Autodesk Inventor part; units mm, degrees
ref_plane "YZ Plane" through (0, 0, 0) normal (1, 0, 0) x (0, 1, 0)
ref_plane "XZ Plane" through (0, 0, 0) normal (0, 1, 0) x (-1, 0, 0)
ref_plane "XY Plane" through (0, 0, 0) normal (0, 0, 1) x (1, 0, 0)
sketch "Sketch1" plane through (0, 0, 0) normal (0, 0, 1) x (1, 0, 0)
  spline S0 degree 3 poles (-37.25, 0) (-37.25, -7.0376) (-35.2039, -14.0633) (-31.4252, -20.0004) (-27.6466, -25.9375) (-22.1482, -30.766) (-15.7726, -33.7459) (-9.397, -36.7258) (-2.1659, -37.8471) (4.8127, -36.9378) (11.7914, -36.0285) (18.4938, -33.0918) (23.893, -28.5778) (29.2921, -24.0637) (33.3697, -17.9875) (35.5009, -11.2804) (37.6321, -4.5732) (37.8097, 2.7422) (36.0064, 9.5448) (34.2031, 16.3475) (30.4251, 22.6143) (25.2512, 27.385) (20.0774, 32.1557) (13.5254, 35.414) (6.5991, 36.6608) (-0.3272, 37.9076) (-7.6042, 37.1385) (-14.1169, 34.4714) (-20.6295, 31.8043) (-26.3557, 27.2483) (-30.4179, 21.5014) (-34.4802, 15.7546) (-36.8647, 8.8365) (-37.2061, 1.8072) (-37.2354, 1.2052) (-37.25, 0.6026) (-37.25, 0) knots 0 0 0 0 0.566787 0.566787 0.566787 1.133573 1.133573 1.133573 1.70036 1.70036 1.70036 2.267146 2.267146 2.267146 2.833933 2.833933 2.833933 3.400719 3.400719 3.400719 3.967506 3.967506 3.967506 4.534292 4.534292 4.534292 5.101079 5.101079 5.101079 5.667865 5.667865 5.667865 6.234652 6.234652 6.234652 6.283185 6.283185 6.283185 6.283185
  spline S1 degree 5 poles (-38.75, 0) (-38.7501, -2.7047) (-38.5078, -5.4094) (-38.0316, -8.0852) (-36.6239, -13.33) (-34.3392, -18.2559) (-32.9845, -20.6148) (-29.8595, -25.0561) (-26.0175, -28.8925) (-23.9357, -30.6396) (-19.4934, -33.7614) (-14.5735, -36.0618) (-12.0149, -36.9831) (-6.7678, -38.3822) (-1.3581, -38.8593) (1.3604, -38.8675) (6.7714, -38.3973) (12.0133, -36.9798) (14.5666, -36.049) (19.4877, -33.7543) (23.9437, -30.6512) (26.0275, -28.9023) (29.8573, -25.0529) (32.972, -20.6052) (34.3321, -18.2523) (36.6385, -13.3362) (38.0403, -8.0889) (38.5046, -5.4103) (38.9743, 0) (38.5079, 5.4103) (38.0448, 8.0901) (36.6331, 13.3345) (34.3305, 18.2516) (32.9714, 20.6051) (29.8608, 25.0551) (26.0293, 28.9037) (23.9413, 30.647) (19.4872, 33.7528) (14.5665, 36.0499) (12.0141, 36.984) (6.7708, 38.3997) (1.3596, 38.8619) (-1.3583, 38.8577) (-6.7678, 38.3823) (-12.0157, 36.988) (-14.5739, 36.063) (-19.4902, 33.7565) (-23.9357, 30.6394) (-26.0178, 28.8927) (-29.8639, 25.0602) (-32.9831, 20.614) (-34.3346, 18.2543) (-36.6237, 13.3303) (-38.0331, 8.0858) (-38.5138, 5.4104) (-38.7506, 2.7047) (-38.75, 0) knots 0 0 0 0 0 0 0.055551 0.055551 0.055551 0.111119 0.111119 0.111119 0.166658 0.166658 0.166658 0.222223 0.222223 0.222223 0.277783 0.277783 0.277783 0.333326 0.333326 0.333326 0.388895 0.388895 0.388895 0.444438 0.444438 0.444438 0.499998 0.499998 0.499998 0.555563 0.555563 0.555563 0.611102 0.611102 0.611102 0.66667 0.66667 0.66667 0.722222 0.722222 0.722222 0.777772 0.777772 0.777772 0.83334 0.83334 0.83334 0.88888 0.88888 0.88888 0.944445 0.944445 0.944445 1 1 1 1 1 1
  spline S2 degree 5 poles (-43.75, 0) (-43.7501, -3.0529) (-43.4775, -6.1058) (-42.9407, -9.1264) (-41.3515, -15.0495) (-38.7703, -20.6121) (-37.2389, -23.2767) (-33.7116, -28.2913) (-29.3743, -32.6225) (-27.0258, -34.5933) (-22.0107, -38.1167) (-16.4569, -40.7135) (-13.5672, -41.7555) (-7.641, -43.3364) (-1.5309, -43.8747) (1.5391, -43.8827) (7.6467, -43.3509) (13.5639, -41.7524) (16.4449, -40.7023) (22.0015, -38.1117) (27.0322, -34.6069) (29.3867, -32.6308) (33.7119, -28.2852) (37.2284, -23.263) (38.763, -20.6081) (41.3648, -15.0583) (42.9484, -9.1357) (43.4738, -6.1111) (44.0049, -0.0005) (43.4774, 6.1102) (42.9529, 9.1371) (41.3593, 15.0572) (38.7607, 20.6082) (37.2277, 23.2632) (33.7158, 28.2869) (29.3897, 32.6312) (27.0312, 34.6016) (22.0016, 38.1099) (16.4443, 40.7036) (13.5628, 41.7573) (7.6441, 43.3536) (1.5365, 43.877) (-1.5313, 43.873) (-7.6403, 43.3367) (-13.5665, 41.7609) (-16.4565, 40.7151) (-22.0073, 38.1119) (-27.0262, 34.5928) (-29.3749, 32.6223) (-33.7159, 28.2954) (-37.237, 23.2766) (-38.7649, 20.6118) (-41.3507, 15.0514) (-42.9418, 9.1288) (-43.4834, 6.1081) (-43.7506, 3.0536) (-43.75, 0) knots 0 0 0 0 0 0 0.055537 0.055537 0.055537 0.111144 0.111144 0.111144 0.166635 0.166635 0.166635 0.222228 0.222228 0.222228 0.277799 0.277799 0.277799 0.333305 0.333305 0.333305 0.388916 0.388916 0.388916 0.444424 0.444424 0.444424 0.499992 0.499992 0.499992 0.555587 0.555587 0.555587 0.611077 0.611077 0.611077 0.666684 0.666684 0.666684 0.722224 0.722224 0.722224 0.777757 0.777757 0.777757 0.833365 0.833365 0.833365 0.888857 0.888857 0.888857 0.944449 0.944449 0.944449 1 1 1 1 1 1
  point P0 (0, 0)
  point P1 (-37.25, 0)
  dimension "d0" = 1.5
  dimension "d1" = 6.5
extrude "Extrusion1" add sketch "Sketch1" against normal blind 40 contours S2
sketch "Sketch5" plane through (0, 0, 0) normal (0, 0, 1) x (1, 0, 0)
  line L0 (-43.75, -6.6095) -> (43.7402, -6.6095)
  line L1 (43.7402, -6.6095) -> (43.7402, 7.3905)
  line L2 (43.7402, 7.3905) -> (-43.75, 7.3905)
  line L3 (-43.75, 7.3905) -> (-43.75, -6.6095)
  line L4 (-43.75, -6.6095) -> (43.7402, 7.3905) construction
  line L5 (43.7402, -6.6095) -> (-43.75, 7.3905) construction
  point P0 (-38.75, 0)
  point P1 (-0.0049, 0.3905)
  dimension "d27" = 14
extrude "Extrusion5" add sketch "Sketch5" along normal blind 5
sketch "Sketch6" plane through (0, 0, 5) normal (0, 0, 1) x (1, 0, 0)
  point P0 (0, 0)
  point P1 (0, 0)
hole "Hole1" at (0, 0, 5) direction (0, 0, -1) diameter 8.5 end through all
properties part number "tunnel"
Build history of the part. All positions in model axes, mm. A direction names the side the tool comes from. Coordinates: 2 decimals unless noted, no trailing zeros.
1. 3-axis set-ups, long thin cutter, end or side, ignore diameter. For faces 4 (the flat face through (-3, 39, 0)), 5 (the flat face through (-1, -6.61, 2)), 6 (the flat face through (43.74, 0, 2)): which of +Z, -Z, +X, -X, +Y, -Y reach the whole face in a straight line?
Answer block:
face 4: +Z, +X, -X, +Y
face 5: +Z, +X, -X, -Y
face 6: +Z, -Z, +X, +Y, -Y
2. Band-saw the part on A-A, the plane x = 7.5. Give the number of separate pieces and of enclosed holes in the cut face, and give its area (3 significant figures).
Answer block:
separate pieces: 3
enclosed holes: 0
area: 477 mm2
3. Drop flat-ended pins along their axis: pin 1 (10 mm diameter, centred on x = 0.5, y = 29.5, fed in from +Z); pin 2 (1 mm diameter, centred on x = 10.5, z = -14, fed in from +Y); pin 3 (3 mm diameter, centred on y = -21.5, z = -30.5, fed in from -X); pin 4 (11 mm diameter, centred on x = 16, y = -2.5, fed in from -Z). Give the stop position or say it passes through.
Answer block:
pin 1: passes through
pin 2: stops at y = 42.59
pin 3: stops at x = -38.91
pin 4: stops at z = 0
4. Pull direction Y, two halves, no side cores. Call faces 1 (the flat face through (1, 7.39, 2)), 2 (the flat face through (3, -39, 0)), 3 (the flat face through (-1, 5, 0)): released by +Y, released by -Y, zero draft, split by the parting line, or undercut.
Answer block:
face 1: released by +Y
face 2: zero draft
face 3: undercut
5. Drill centre lines: probe 1 along X at (y, z) = (0, 1.45); probe 2 along Y at (x, z) = (0, 2.95); probe 3 along Y at (x, z) = (24.5, 1.5). Where is each one in solid material? Low to high.
Answer block:
probe 1: x = -43.75 to -4.25, 4.25 to 43.74
probe 2: y = -6.61 to -4.25, 4.25 to 7.39
probe 3: y = -6.61 to 7.39
